Read the model definition and answer for the solid it produces. Units are mm, in the model's axes. A direction names the side the tool comes from. Round coordinates to 2 decimals unless told otherwise and drop trailing zeros. Write each loop counter-clockwise with the first axis right and the second up, starting at its lowest first coordinate (ties: lowest second). Pieces come first, ordered by that corner, then holes. Notation, with made-up numbers: (-5.75, 25) - (-1.75, 25) arc R27 ccw to (-1.75, 44) - close; hole circle Ø8 at (83, 81.25). An arc over 180 degrees is marked (long way). One line per item, written item: value. Start each with the question number.
(1) Find the intervals of material crossed by L1, parallel to Z at x = -4.5, y = 2.5; L2, parallel to Y at x = -9.75, z = -17.5; L3, parallel to Y at x = -9.5, z = -32.5, in increasing order.
(2) A cutting plane is placed at B-B, the plane z = -33. Determine the outline of the cut face in (x, y), plus the area to 3 significant figures.
(3) A cutting plane is placed at D-D, the plane x = -3.75. Determine the outline of the cut face in (y, z).
(4) The mould has two halves that part along Z. Classify faces 1 (the face through (-5, -3, -29.75)), 2 (the face through (-7.2, 1.6, -23.7)), 3 (the face through (-6.9, 2, -41)): +Z half, -Z half, draft (parallel to the pull), parting line (faces both ways), or undercut.
(5) A cutting plane is placed at C-C, the plane y = -1.5. Determine the outline of the cut face in (x, z), plus the area to 4 significant figures.
(6) For faces 4 (the face through (1, 0, -32)), 5 (the face through (-3.1, 2, -7)), 6 (the face through (-5, 2.98, -24)), 7 (the face through (-5, 2, -31.2)), determine the directions among +Z, -Z, +X, -X, +Y, -Y from which every point of the face is accessible in a straight line to the end or side of a thin tool.
(7) Flat-ended cylindrical pins translate along their axes: pin 1 Ø1.6 at (x, y) = (-5.5, 2.5) entering from +Z; pin 2 Ø3 at (x, z) = (-4.5, -27) entering from +Y; pin 3 Ø8 at (x, z) = (-6.5, -41.5) entering from -Y. Find the tip coordinate at first contact, or state that the pin passes through.
(8) A cutting plane is placed at A-A, the plane x = -9. Determine the outline of the cut face in (y, z).
Autodesk Inventor part; units mm, degrees
ref_plane "YZ Plane" through (0, 0, 0) normal (1, 0, 0) x (0, 1, 0)
ref_plane "XZ Plane" through (0, 0, 0) normal (0, 1, 0) x (-1, 0, 0)
ref_plane "XY Plane" through (0, 0, 0) normal (0, 0, 1) x (1, 0, 0)
sketch "Sketch2" plane through (0, 0, 0) normal (0, 1, 0) x (-1, 0, 0)
  line L0 (10, 0) -> (0, 0)
  line L1 (0, 0) -> (0, -48)
  line L2 (0, -48) -> (10, -48)
  line L3 (10, -48) -> (10, 0)
  line L4 (6.9, -8.3) -> (3.1, -8.3)
  line L5 (3.1, -8.3) -> (3.1, -5.7)
  line L6 (3.1, -5.7) -> (6.9, -5.7)
  line L7 (6.9, -5.7) -> (6.9, -8.3)
  line L8 (6.9, -39.7) -> (3.1, -39.7)
  line L9 (3.1, -39.7) -> (3.1, -42.3)
  line L10 (3.1, -42.3) -> (6.9, -42.3)
  line L11 (6.9, -42.3) -> (6.9, -39.7)
  line L12 (3.1, -22.7) -> (6.9, -22.7)
  line L13 (3.1, -25.3) -> (3.1, -22.7)
  line L14 (6.9, -25.3) -> (3.1, -25.3)
  line L15 (6.9, -22.7) -> (6.9, -25.3)
  line L16 (23.6892, -32.5) -> (-2.3247, -32.5) construction
  line L17 (5, -54.7987) -> (5, -48.1542) construction
  line L18 (5, 9.3713) -> (5, -46.1174) construction
  line L19 (11.7769, -7) -> (1.25, -7) construction
  line L20 (11.7769, -24) -> (1.25, -24) construction
  line L21 (11.7769, -41) -> (1.25, -41) construction
  line L22 (12.75, -29.75) -> (-2.75, -29.75)
  line L23 (-2.75, -35.25) -> (12.75, -35.25)
  line L24 (12.75, -29.75) -> (12.75, -35.25)
  line L25 (-2.75, -29.75) -> (-2.75, -35.25)
  dimension "d0" = 10
  dimension "d1" = 48
  dimension "d13" = 3.8
  dimension "d14" = 2.6
  dimension "d40" = 5
  dimension "d49" = 15.5
  dimension "d50" = 7
  dimension "d51" = 24
  dimension "d52" = 41
  dimension "d53" = 5.5
  dimension "d54" = 15.5
extrude "Extrusion1" add sketch "Sketch2" along normal blind 1.6 contours L3 L22 L1 L0 | L3 L23 L1 L22 | L3 L2 L1 L23 | L4 L5 L6 L7 | L11 L10 L9 L8 | L12 L15 L14 L13
extrude "Extrusion4" add sketch "Sketch2" along normal blind 2.98 contours L4 L5 L6 L7 | L11 L10 L9 L8 | L12 L15 L14 L13
sketch "Sketch3" plane through (0, 2.98, 0) normal (0, 1, 0) x (1, 0, 0)
  line L0 (-3.1, 25.3) -> (-6.9, 25.3) construction
  line L1 (-6.9, 22.7) -> (-3.1, 22.7) construction
  point P0 (0, 0)
  point P1 (-5.1459, 24.0493)
extrude "Extrusion5" add sketch "Sketch2" against normal blind 5.5 contours L22 L24 L23 L3 | L3 L23 L1 L22 | L1 L23 L25 L22
sketch "Sketch4" plane through (0, 1.6, 0) normal (0, 1, 0) x (1, 0, 0)
  line L0 (-1.75, 31.2) -> (-8.25, 31.2)
  line L1 (-8.25, 31.2) -> (-8.25, 33.8)
  line L2 (-8.25, 33.8) -> (-1.75, 33.8)
  line L3 (-1.75, 33.8) -> (-1.75, 31.2)
  line L4 (-23.6892, 32.5) -> (2.3247, 32.5) construction
  line L5 (-5, -9.3713) -> (-5, 46.1174) construction
  point P0 (0, 0)
  dimension "d57" = 2.6
  dimension "d58" = 6.5
extrude "Extrusion6" add sketch "Sketch4" along normal blind 1.5
properties part number "Sensor_Board_dummy"
Here are the results:
1. L1: -42.3 to -39.7, -33.8 to -31.2, -25.3 to -22.7, -8.3 to -5.7
1. L2: 0 to 1.6
1. L3: -5.5 to 1.6
2. outline: (-12.75, -5.5) - (2.75, -5.5) - (2.75, 0) - (0, 0) - (0, 1.6) - (-1.75, 1.6) - (-1.75, 3.1) - (-8.25, 3.1) - (-8.25, 1.6) - (-10, 1.6) - (-10, 0) - (-12.75, 0) - close
2. area: 111 mm²
3. outline: (-5.5, -35.25) - (0, -35.25) - (0, -48) - (1.6, -48) - (1.6, -42.3) - (2.98, -42.3) - (2.98, -39.7) - (1.6, -39.7) - (1.6, -33.8) - (3.1, -33.8) - (3.1, -31.2) - (1.6, -31.2) - (1.6, -25.3) - (2.98, -25.3) - (2.98, -22.7) - (1.6, -22.7) - (1.6, -8.3) - (2.98, -8.3) - (2.98, -5.7) - (1.6, -5.7) - (1.6, 0) - (0, 0) - (0, -29.75) - (-5.5, -29.75) - close
4. face 1: +Z half
4. face 2: undercut
4. face 3: draft
5. outline: (-12.75, -35.25) - (2.75, -35.25) - (2.75, -29.75) - (-12.75, -29.75) - close
5. area: 85.25 mm²
6. face 4: +Z, -Z, +X, +Y
6. face 5: +Z, +X, +Y
6. face 6: +Z, +X, -X, +Y
6. face 7: +X, -X, +Y
7. pin 1: z = -5.7
7. pin 2: y = 1.6
7. pin 3: y = 0
8. outline: (-5.5, -35.25) - (0, -35.25) - (0, -48) - (1.6, -48) - (1.6, 0) - (0, 0) - (0, -29.75) - (-5.5, -29.75) - close
